from build123d import *

# Parameters (mm, degrees)
SKETCH1_W           = 79
SKETCH1_H           = 68.072
BOSS_EXTRUDE1_DEPTH = 0.5
FILLET1_R           = 4
CUT_EXTRUDE1_DEPTH  = 53.143545104


with BuildPart() as part:
    # Sketch1 → Boss-Extrude1 (new body)
    with BuildSketch(Plane.XY):
        Rectangle(SKETCH1_W, SKETCH1_H)
    extrude(amount=BOSS_EXTRUDE1_DEPTH)

    # Fillet1
    fillet1_edges = [part.edges().sort_by_distance(p)[0] for p in [
        (-39.5, 34.036, 0.25),
        (39.5, 34.036, 0.25),
        (39.5, -34.036, 0.25),
        (-39.5, -34.036, 0.25),
    ]]
    fillet(fillet1_edges, radius=FILLET1_R)

    # Sketch2 → Cut-Extrude1 (cut, through all)
    with BuildSketch(Plane.XY.offset(0.5)):
        with BuildLine():
            Line((-19.428, 16.002), (30.864, 16.002))
            ThreePointArc((30.864, 16.002), (32.480446102, 15.332446102), (33.15, 13.716))
            Line((33.15, 13.716), (33.15, -13.462))
            ThreePointArc((33.15, -13.462), (32.480446102, -15.078446102), (30.864, -15.748))
            Line((30.864, -15.748), (-19.428, -15.748))
            ThreePointArc((-19.428, -15.748), (-21.044446102, -15.078446102), (-21.714, -13.462))
            Line((-21.714, -13.462), (-21.714, 13.716))
            ThreePointArc((-21.714, 13.716), (-21.044446102, 15.332446102), (-19.428, 16.002))
        make_face()
    extrude(amount=-CUT_EXTRUDE1_DEPTH, mode=Mode.SUBTRACT)


solid = part.part
Can you work these out from the model? Positions are in its coordinate system, mm. A direction names the side the tool comes from. Round coordinates to 2 decimals unless told otherwise and drop trailing zeros. Loops run counter-clockwise (first coordinate to the right, second up) from the corner with the lowest first, then second, coordinate; pieces in that order, holes last. Notation, with made-up numbers: (67, -9) - (103, -9) arc R34 ccw to (103, 23) - close; hole circle Ø7 at (-19.5, 39.5). An arc over 180 degrees is marked (long way). Write item = value, one per line. Start each with the question number.
(1) If we section it at B-B (y = -12.5): Please give me the cut outline in (x, z), and give its area (3 significant figures).
(2) If we section it at A-A (x = 26): Please give me the cut outline in (y, z), and give its area (3 significant figures).
(3) If we mould it in two halves opening along X, with no side actions, what happens to faces 1 (the face through (32.5, -15.06, 0.25)), 2 (the face through (-38.36, 32.83, 0.25)), 3 (the face through (-1, 23, 0.5))? For each: released by +X, released by -X, zero draft, split by the parting line, or undercut.
(4) If we section it at C-C (z = 0.15): Please give me the cut outline in (x, y), and give its area (3 significant figures).
(5) For faces 4 (the face through (32.46, 15.35, 0.25)), 5 (the face through (38.297, -32.895, 0.254)), which set-ups out of +Z, -Z, +X, -X, +Y, -Y let a thin tool reach every point of the face, with its end or its side?
(6) If I drill on probe 1 along Y at (x, z) = (20.5, 0.45); probe 2 along X at (y, z) = (-1, 0.2), over which ranges is the centre line in solid material (lowest first)? Write a range as [from, to].
Ans:
q1.outline = (-39.5, 0) - (-21.71, 0) - (-21.71, 0.5) - (-39.5, 0.5) - close; (33.15, 0) - (39.5, 0) - (39.5, 0.5) - (33.15, 0.5) - close
q1.area = 12.1 mm²
q2.outline = (-34.04, 0) - (-15.75, 0) - (-15.75, 0.5) - (-34.04, 0.5) - close; (16, 0) - (34.04, 0) - (34.04, 0.5) - (16, 0.5) - close
q2.area = 18.2 mm²
q3.face_1 = undercut
q3.face_2 = released by -X
q3.face_3 = zero draft
q4.outline = (-39.5, -30.04) arc R4 ccw to (-35.5, -34.04) - (35.5, -34.04) arc R4 ccw to (39.5, -30.04) - (39.5, 30.04) arc R4 ccw to (35.5, 34.04) - (-35.5, 34.04) arc R4 ccw to (-39.5, 30.04) - close; hole (-21.71, -13.46) arc R2.29 ccw to (-19.43, -15.75) - (30.86, -15.75) arc R2.29 ccw to (33.15, -13.46) - (33.15, 13.72) arc R2.29 ccw to (30.86, 16) - (-19.43, 16) arc R2.29 ccw to (-21.71, 13.72) - close
q4.area = 3,630 mm²
q5.face_4 = +Z, -Z
q5.face_5 = +Z, -Z, +X, -Y
q6.probe_1 = [-34.04, -15.75], [16, 34.04]
q6.probe_2 = [-39.5, -21.71], [33.15, 39.5]
